from build123d import *

# Parameters (mm, degrees)
F2_DEPTH     = 2.5
F3_DEPTH     = 10
F4_DEPTH     = 3
F5_DEPTH     = 6
F6_T1_DEPTH  = 5
F8_DEPTH     = 14
F9_DEPTH     = 9
F10_DEPTH    = 1
F11_DEPTH    = 16.5
F12_T4_DEPTH = 5
F14_DEPTH    = 6
F15_T1_DEPTH = 35.9238558823


# Not quite as in the source:
# - a fillet or chamfer that OpenCascade refuses, or shapes differently, is made with other operations: its cross-section is extruded or revolved along the edge and cut away or added


with BuildPart() as f2:
    # F0 (on Front) → F2 (new body, symmetric)
    with BuildSketch(Plane.XZ):
        Polygon((0, 3.5), (0, 0), (9, 0), (9, 14), (6, 14), (6, 3.5), align=None)
    extrude(amount=F2_DEPTH, both=True)

    # F1 (on Right) → F3 (join)
    with BuildSketch(Plane.YZ):
        with BuildLine():
            Line((-2.5, 14), (2.5, 14))
            ThreePointArc((2.5, 14), (0, 16.5), (-2.5, 14))
        make_face()
        with BuildLine():
            ThreePointArc((-2.5, 14), (0, 11.5), (2.5, 14))
            Line((2.5, 14), (-2.5, 14))
        make_face()
    extrude(amount=F3_DEPTH)

    # F1 (on Right) → F4 (cut)
    with BuildSketch(Plane.YZ):
        with BuildLine():
            Line((-2.5, 14), (2.5, 14))
            ThreePointArc((2.5, 14), (0, 16.5), (-2.5, 14))
        make_face()
        with BuildLine():
            ThreePointArc((-2.5, 14), (0, 11.5), (2.5, 14))
            Line((2.5, 14), (-2.5, 14))
        make_face()
    extrude(amount=F4_DEPTH, mode=Mode.SUBTRACT)

    # F1 (on Right) → F5 (cut)
    with BuildSketch(Plane.YZ):
        with BuildLine():
            ThreePointArc((-2.5, 14), (0, 11.5), (2.5, 14))
            Line((2.5, 14), (-2.5, 14))
        make_face()
    extrude(amount=F5_DEPTH, mode=Mode.SUBTRACT)

    # F6: fillet of radius 1 on 2 edges, made by hand

    # F6_s2 → F6_t1 (join)
    with BuildSketch(Plane.XZ.offset(-2.5)):
        with BuildLine():
            ThreePointArc((6, 13), (5.7071067812, 13.7071067812), (5, 14))
            Line((5, 14), (6, 14))
            Line((6, 14), (6, 13))
        make_face()
        with BuildLine():
            ThreePointArc((5, 3.5), (5.7071067812, 3.7928932188), (6, 4.5))
            Line((6, 4.5), (6, 3.5))
            Line((6, 3.5), (5, 3.5))
        make_face()
    extrude(amount=F6_T1_DEPTH)

    # F7 (on Top) → F8 (join)
    with BuildSketch(Plane.XY):
        Polygon((9, 2.5), (9, -2.5), (10, 0), align=None)
    extrude(amount=F8_DEPTH)

    # F7 (on Top) → F9 (cut)
    with BuildSketch(Plane.XY):
        Polygon((9, 2.5), (9, -2.5), (10, 0), align=None)
    extrude(amount=F9_DEPTH, mode=Mode.SUBTRACT)

    # F10 (add): a face of the model
    f10_faces = [f2.faces().sort_by_distance(p)[0] for p in [
        (10, -1.717766953, 12.282233047),
    ]]
    extrude(f10_faces, amount=F10_DEPTH)

    # F7 (on Top) → F11 (cut)
    with BuildSketch(Plane.XY):
        Polygon((11, 0), (10, -2.5), (11.5, -2.5), (11.5, 2.5), (10, 2.5), align=None)
    extrude(amount=F11_DEPTH, mode=Mode.SUBTRACT)

    # F12: chamfer of 1 x 5.6712818196 on 1 edges, made by hand


with BuildPart() as f12_tool2:
    # F12_s3 → F12_t4 (new body)
    with BuildSketch(Plane.XZ.offset(-2.5)):
        Polygon((10, 9), (9, 3.3287181804), (9, 9), align=None)
    extrude(amount=F12_T4_DEPTH)

    split(bisect_by=Plane(origin=(8.6206896552, 3.4482758621, 0), x_dir=(0, 0, 1), z_dir=(-0.9284766909, -0.3713906764, 0)), keep=Keep.TOP)

    split(bisect_by=Plane(origin=(8.6206896552, -3.4482758621, 0), x_dir=(0, 0, 1), z_dir=(-0.9284766909, 0.3713906764, 0)), keep=Keep.TOP)


with BuildPart() as f2_1:
    add(f2.part)

    # F12_t1: union F12_tool2
    add(f12_tool2.part)

    # F13: F2 across face


with BuildPart() as f2_2:
    add(f2_1.part)
    add(f2_1.part.mirror(Plane(origin=(0, 0, 1.75), x_dir=(0, -1, 0), z_dir=(-1, 0, 0))))

    # F14 (add): a face of the model
    f14_faces = [f2_2.faces().sort_by_distance(p)[0] for p in [
        (0, 0, 0),
    ]]
    extrude(f14_faces, amount=F14_DEPTH)

    # F15: chamfer of 2 x 3.4641016151 on 2 edges, made by hand

    # F15_s2 → F15_t1 (cut)
    with BuildSketch(Plane.YZ.offset(-17.9619279412)):
        Polygon((-2.5, -4), (0.9641016151, -6), (-2.5, -6), align=None)
        Polygon((-0.9641016151, -6), (2.5, -4), (2.5, -6), align=None)
    extrude(amount=F15_T1_DEPTH, mode=Mode.SUBTRACT)


solid = f2_2.part
Can you work these out from the model? Positions are in its coordinate system, mm. A direction names the side the tool comes from. Give positions to 0.01 mm unless a question says otherwise; leave off trailing zeros. Loops run counter-clockwise (first coordinate to the right, second up) from the corner with the lowest first, then second, coordinate; pieces in that order, holes last. Notation, with made-up numbers: (8, 56) -> (59, 56) arc R25 ccw to (59, 74) -> close; hole circle Ø6 at (2, 2). An arc over 180 degrees is marked (long way). Return JSON: item names as keys, results as strings.
Q1. I want a section at A-A, the plane z = 10.5. List the corners of the cut face in (x, y) for me.
Checks:
{"outline": "(-10, 0) -> (-9, -2.5) -> (-6, -2.5) -> (-6, 2.5) -> (-9, 2.5) -> close; (6, -2.5) -> (9, -2.5) -> (10, 0) -> (9, 2.5) -> (6, 2.5) -> close"}
Q2. On a 3-axis mill with a long thin cutter (end or side, diameter ignored), from which of +Z, -Z, +X, -X, +Y, -Y can I reach the whole of each face in a straight line? I mean faces 1 (the face through (3, 0, 15)), 2 (the face through (-9, 0, -1)), 3 (the face through (-0.126, 1.233, -4.732)), 4 (the face through (4, 0, 14)), 5 (the face through (-0.13, -1.27, -4.71)). Say none if no direction works.
Checks:
{"face 1": "+Z, +Y, -Y", "face 2": "-Z, -X, +Y, -Y", "face 3": "-Z, +X, -X, +Y", "face 4": "+Y, -Y", "face 5": "-Z, +X, -X, -Y"}
Q3. I need wall thicknesses on probe 1 along X at (y, z) = (0.1, 0.5); probe 2 along X at (y, z) = (-1.4, 6.75); probe 3 along X at (y, z) = (1.85, 9). Which ranges of each line are inside material? Lowest first, please.
Checks:
{"probe 1": "x = -9 to 9", "probe 2": "x = -9.44 to -6, 6 to 9.44", "probe 3": "x = -9.26 to -6, 6 to 9.26"}
Q4. I want a section at D-D, the plane y = 1.5. List the corners of the cut face in (x, z) for me, then the cut area to 3 significant figures.
Checks:
{"outline": "(-10.4, 12) -> (-9.4, 12) -> (-9.4, 5.6) -> (-9, 3.33) -> (-9, -4.58) -> (9, -4.58) -> (9, 3.33) -> (9.4, 5.6) -> (9.4, 12) -> (10.4, 12) -> (10.4, 16) -> (3, 16) -> (3, 14) -> (5, 14) arc R1 cw to (6, 13) -> (6, 4.5) arc R1 cw to (5, 3.5) -> (-5, 3.5) arc R1 cw to (-6, 4.5) -> (-6, 13) arc R1 cw to (-5, 14) -> (-3, 14) -> (-3, 16) -> (-10.4, 16) -> close", "area": "250 mm2"}
Q5. For pin 1 Ø1.2 at (y, z) = (1, 15.5) entering from -X; pin 2 Ø2 at (x, y) = (4, 0.5) entering from -Z; pin 3 Ø1.5 at (x, y) = (0.5, -0.5) entering from +Z, each with a flat end and sliding along its axis, tell me the tip position at first contact or that it passes through.
Checks:
{"pin 1": "stops at x = -10.84", "pin 2": "stops at z = -5.44", "pin 3": "stops at z = 3.5"}
Q6. I want a section at C-C, the plane z = 0. List the corners of the cut face in (x, y) for me, then the cut area to 3 significant figures.
Checks:
{"outline": "(-9, -2.5) -> (9, -2.5) -> (9, 2.5) -> (-9, 2.5) -> close", "area": "90.0 mm2"}
Q7. I want a section at B-B, the plane y = -1.65. List the corners of the cut face in (x, z) for me, then the cut area to 3 significant figures.
Checks:
{"outline": "(-10.34, 12.12) -> (-9.34, 12.12) -> (-9.34, 5.26) -> (-9, 3.33) -> (-9, -4.49) -> (9, -4.49) -> (9, 3.33) -> (9.34, 5.26) -> (9.34, 12.12) -> (10.34, 12.12) -> (10.34, 15.88) -> (3, 15.88) -> (3, 14) -> (5, 14) arc R1 cw to (6, 13) -> (6, 4.5) arc R1 cw to (5, 3.5) -> (-5, 3.5) arc R1 cw to (-6, 4.5) -> (-6, 13) arc R1 cw to (-5, 14) -> (-3, 14) -> (-3, 15.88) -> (-10.34, 15.88) -> close", "area": "246 mm2"}
